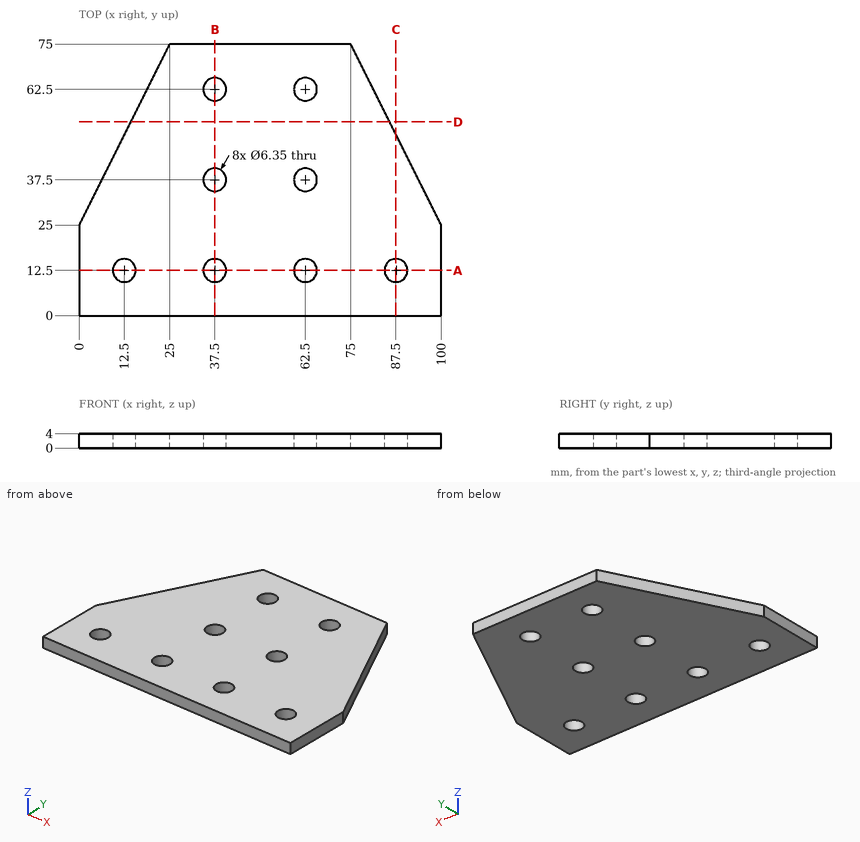
Geometry check sheet. Reference: drawing and pictorial views, mm from the part's lowest x, y, z. Round coordinates to 2 decimals unless told otherwise and drop trailing zeros. Loops run counter-clockwise (first coordinate to the right, second up) from the corner with the lowest first, then second, coordinate; pieces in that order, holes last. Notation, with made-up numbers: (-18.75, 41) - (19.25, 41) arc R16 cw to (19.25, 62) - close; hole circle Ø2 at (2, -2.75). An arc over 180 degrees is marked (long way). One line per question, with ' | ' between items. Start each with the question number.
1. Depth check by flat-ended pin: pin 1 (1 mm diameter, centred on y = 65.5, z = 3, fed in from +X); pin 2 (1 mm diameter, centred on y = 63, z = 1, fed in from -X). Enter the tip coordinate at first touch or a pass-through.
2. Cross-section at B-B on x = 37.5. Record the cut outline in (y, z) (3 decimals), then the cut area to 3 significant figures.
3. Cross-section at A-A on y = 12.5. Record the cut outline in (x, z) (3 decimals), then the cut area to 3 significant figures.
4. Cross-section at D-D on y = 53.5. Record the cut outline in (x, z), then the cut area to 3 significant figures.
5. Cross-section at C-C on x = 87.5. Record the cut outline in (y, z) (3 decimals).
6. Scan lines: line 1 (Y direction, x = 37.5, z = 2.5) (3 decimals); line 2 (X direction, y = 35.5, z = 2.5); line 3 (X direction, y = 36, z = 2.55). Record each from-to range of solid material in increasing order. Write a range as [from, to].
Taken from the geometry:
1) pin 1: x = 80 | pin 2: x = 18.75
2) outline: (0, 0) - (9.325, 0) - (9.325, 4) - (0, 4) - close; (15.675, 0) - (34.325, 0) - (34.325, 4) - (15.675, 4) - close; (40.675, 0) - (59.325, 0) - (59.325, 4) - (40.675, 4) - close; (65.675, 0) - (75, 0) - (75, 4) - (65.675, 4) - close | area: 224 mm²
3) outline: (0, 0) - (9.325, 0) - (9.325, 4) - (0, 4) - close; (15.675, 0) - (34.325, 0) - (34.325, 4) - (15.675, 4) - close; (40.675, 0) - (59.325, 0) - (59.325, 4) - (40.675, 4) - close; (65.675, 0) - (84.325, 0) - (84.325, 4) - (65.675, 4) - close; (90.675, 0) - (100, 0) - (100, 4) - (90.675, 4) - close | area: 298 mm²
4) outline: (14.25, 0) - (85.75, 0) - (85.75, 4) - (14.25, 4) - close | area: 286 mm²
5) outline: (0, 0) - (9.325, 0) - (9.325, 4) - (0, 4) - close; (15.675, 0) - (50, 0) - (50, 4) - (15.675, 4) - close
6) line 1: [0, 9.325], [15.675, 34.325], [40.675, 59.325], [65.675, 75] | line 2: [5.25, 35.03], [39.97, 60.03], [64.97, 94.75] | line 3: [5.5, 34.7], [40.3, 59.7], [65.3, 94.5]
